Here's how the part is built. I have some questions about the finished solid (model axes, mm). A direction names the side the tool comes from. Give positions to 0.01 mm unless a question says otherwise; leave off trailing zeros. Loops run counter-clockwise (first coordinate to the right, second up) from the corner with the lowest first, then second, coordinate; pieces in that order, holes last. Notation, with made-up numbers: (33.25, -31) -> (78.25, -31) arc R29 cw to (78.25, 1) -> close; hole circle Ø7 at (85.5, -27). An arc over 180 degrees is marked (long way). Answer in a Markdown table with one row per item. Add a question column.
Item 1: We'd pull the mould along Y, two halves only. Please class faces 4 (the face through (-1.1, -1, 2)), 5 (the face through (1.25, -0.9, 2.5)), 6 (the face through (0, -3, 0)): released by +Y, released by -Y, zero draft, split by the parting line, or undercut.
Item 2: If we section it at C-C (x = -0.8): Write out the boundary of the cut face in (y, z), then the cut area to 3 significant figures.
Item 3: If we section it at D-D (y = 3.25): Write out the boundary of the cut face in (x, z).
Item 4: For P1, Ø1, axis at x = -0.5, z = -1.5, coming from the +Y side; P2, Ø1.5, axis at y = -1, z = 1, coming from the -X side, each with a flat end and sliding along its axis, tell me the tip position at first contact or that it passes through.
Item 5: Which directions (+Z, -Z, +X, -X, +Y, -Y) give clear straight access to the entire face, cutting with the end or side of a thin tool? Please do faces 1 (the face through (0.954, 3.434, 1.081)), 2 (the face through (0.65, -1, 3)), 3 (the face through (1.1, -1, 2)).
Item 6: If I drill on line 1 (Z direction, x = -1.15, y = 0); line 2 (Z direction, x = -1.05, y = 0); line 3 (Z direction, x = 1.2, y = 0), over which ranges is the centre line in solid material (lowest first)?
Autodesk Inventor part; units mm, degrees
ref_plane "YZ Plane" through (0, 0, 0) normal (1, 0, 0) x (0, 1, 0)
ref_plane "XZ Plane" through (0, 0, 0) normal (0, 1, 0) x (-1, 0, 0)
ref_plane "XY Plane" through (0, 0, 0) normal (0, 0, 1) x (1, 0, 0)
sketch "_____1" plane through (0, 0, 0) normal (0, 0, 1) x (1, 0, 0)
  line L0 (50, 0) -> (-50, 0)
  line L1 (-1.25, 0) -> (-1.25, 2)
  line L2 (-1.25, 2) -> (-1.1, 2)
  line L3 (-1.1, 2) -> (-1.1, 2.5)
  line L4 (-1.1, 2.5) -> (-1.25, 2.5)
  line L5 (-1.25, 2.5) -> (-1.25, 2.9)
  arc A0 (-1.15, 3) -> (-1.25, 2.9) centre (-1.15, 2.9) ccw
  line L6 (-1.15, 3) -> (0.65, 3)
  line L7 (0.65, 3) -> (0.65, 3.6)
  line L8 (0.65, 3.6) -> (1.25, 3.6)
  line L9 (1.25, 3.6) -> (1.25, 2.5)
  line L10 (1.25, 2.5) -> (1.1, 2.5)
  line L11 (1.1, 2.5) -> (1.1, 2)
  line L12 (1.1, 2) -> (1.25, 2)
  line L13 (1.25, 2) -> (1.25, 0)
  line L14 (1.25, 0) -> (-1.25, 0)
revolve "Revolution1" add sketch "_____1" angle 360 about axis through (50, 0, 0) along (1, 0, 0)
sketch "_____2" plane through (0, 0, 0) normal (0, 0, 1) x (1, 0, 0)
  line L0 (50, 0) -> (-50, 0)
  line L1 (-1.25, 0) -> (-1.25, 1.6)
  arc A0 (-1.25, 1.6) -> (-1.15, 1.5) centre (-1.15, 1.6) ccw
  line L2 (-1.15, 1.5) -> (1.15, 1.5)
  arc A1 (1.15, 1.5) -> (1.25, 1.6) centre (1.15, 1.6) ccw
  line L3 (1.25, 1.6) -> (1.25, 0)
  line L4 (1.25, 0) -> (-1.25, 0)
revolve "Revolution2" cut sketch "_____2" angle 360 about axis through (50, 0, 0) along (1, 0, 0)
properties part number "C-FL673ZZ"
Recorded:
| question | item | result |
|---|---|---|
| 1 | face 4 | undercut |
| 1 | face 5 | zero draft |
| 1 | face 6 | split by the parting line |
| 2 | outline | circle Ø6 at (0, 0); hole circle Ø3 at (0, 0) |
| 2 | area | 21.2 mm^2 |
| 3 | outline | (0.65, -1.55) -> (1.25, -1.55) -> (1.25, 1.55) -> (0.65, 1.55) -> close |
| 4 | P1 | stops at y = 2.83 |
| 4 | P2 | stops at x = -1.25 |
| 5 | face 1 | +X, -X |
| 5 | face 2 | -X |
| 5 | face 3 | +X |
| 6 | line 1 | z = -3 to -2.5, -2 to -1.5, 1.5 to 2, 2.5 to 3 |
| 6 | line 2 | z = -3 to -1.5, 1.5 to 3 |
| 6 | line 3 | z = -3.6 to -2.5, -2 to -1.51, 1.51 to 2, 2.5 to 3.6 |
